The drawing under review shows one solid part. Ordinate dimensions are in mm from its lowest x, y, z. A direction names the side the tool comes from. Coordinates: 2 decimals unless noted, no trailing zeros. Loops run counter-clockwise (first coordinate to the right, second up) from the corner with the lowest first, then second, coordinate; pieces in that order, holes last. Notation, with made-up numbers: M 65.5,-34.75 L 93.5,-34.75 A29 ccw 93.5,-10.75 Z; hole C 41.5,76 d11. An arc over 180 degrees is marked long. Answer as CSV lines item,"result". Start each with the question number.
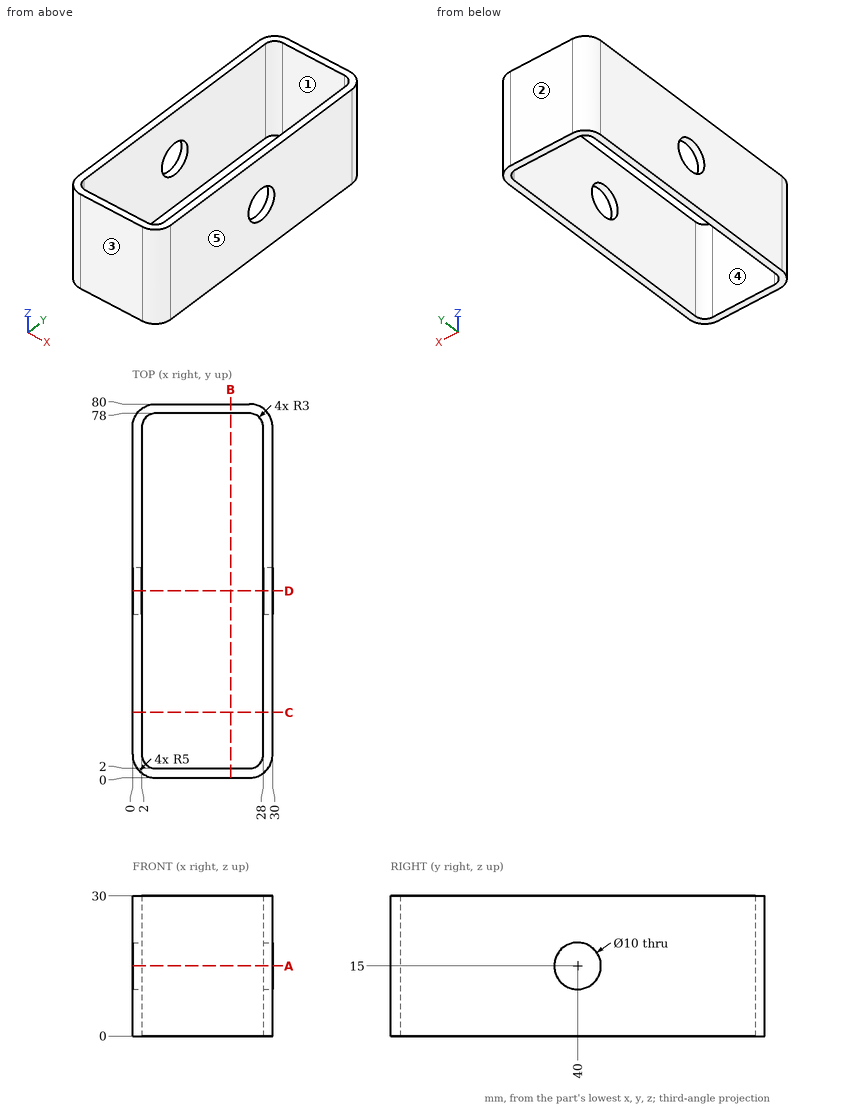
Item 1: For line 1 along Z through (x, y) = (28.95, 40); line 2 along X through (y, z) = (9, 22.5); line 3 along Y through (x, z) = (14.75, 11.75), list the stretches that pass through material, from the lowest coordinate up. Write a range as from..to.
Item 2: Mouldability with a two-part tool opening along X and no side actions: class the marked faces 3, 4 and 5 as released by +X, released by -X, zero draft, split by the parting line, or undercut.
Item 3: Add section D-D (y = 40). Give the boundary of the cut face in (x, z), plus the area to 3 significant figures.
Item 4: Add section B-B (x = 21). Give the boundary of the cut face in (y, z).
Item 5: Add section A-A (z = 15). Give the boundary of the cut face in (x, y).
Item 6: For the marked faces 1 and 2, list the 3-axis set-ups (+Z, -Z, +X, -X, +Y, -Y) from which the entire face can be reached by the end or side of a thin tool; tool diameter is ignored.
Item 7: Add section C-C (y = 14). Give the boundary of the cut face in (x, z), plus the area to 3 significant figures.
Response:
1,line 1,"0..10, 20..30"
1,line 2,"0..2, 28..30"
1,line 3,"0..2, 78..80"
2,face 3,"zero draft"
2,face 4,"undercut"
2,face 5,"released by +X"
3,outline,"M 0,0 L 2,0 L 2,10 L 0,10 Z; M 0,20 L 2,20 L 2,30 L 0,30 Z; M 28,0 L 30,0 L 30,10 L 28,10 Z; M 28,20 L 30,20 L 30,30 L 28,30 Z"
3,area,"80.0 mm²"
4,outline,"M 0,0 L 2,0 L 2,30 L 0,30 Z; M 78,0 L 80,0 L 80,30 L 78,30 Z"
5,outline,"M 0,5 A5 ccw 5,0 L 25,0 A5 ccw 30,5 L 30,35 L 28,35 L 28,5 A3 cw 25,2 L 5,2 A3 cw 2,5 L 2,35 L 0,35 Z; M 0,45 L 2,45 L 2,75 A3 cw 5,78 L 25,78 A3 cw 28,75 L 28,45 L 30,45 L 30,75 A5 ccw 25,80 L 5,80 A5 ccw 0,75 Z"
6,face 1,"+Z, -Z"
6,face 2,"+Z, -Z, +X, -X, +Y"
7,outline,"M 0,0 L 2,0 L 2,30 L 0,30 Z; M 28,0 L 30,0 L 30,30 L 28,30 Z"
7,area,"120 mm²"
